from build123d import *

# Parameters (mm, degrees)
F1_DEPTH = 25.4
F2_R     = 3.175
F3_DEPTH = 25.4
F4_T     = -2.54


with BuildPart() as f1:
    # F0 (on Front) → F1 (new body)
    with BuildSketch(Plane.XZ):
        with BuildLine():
            Line((-63.5, -38.1), (63.5, -38.1))
            Line((63.5, -38.1), (63.5, 3.0236337334))
            Line((63.5, 3.0236337334), (6.35, 38.1))
            Line((6.35, 38.1), (-50.8, 38.1))
            ThreePointArc((-50.8, 38.1), (-59.7802561211, 34.3802561211), (-63.5, 25.4))
            Line((-63.5, 25.4), (-63.5, -38.1))
        make_face()
    extrude(amount=F1_DEPTH)

    # F2 (on face) → F3 (cut)
    with BuildSketch(Plane.XZ.offset(25.4)):
        with Locations((-50.8, 25.4)):
            Circle(F2_R)
        with Locations((-50.8, 0)):
            Circle(F2_R)
        with Locations((-50.8, -25.4)):
            Circle(F2_R)
        with Locations((-38.1, 25.4)):
            Circle(F2_R)
        with Locations((-38.1, 0)):
            Circle(F2_R)
        with Locations((-38.1, -25.4)):
            Circle(F2_R)
        with Locations((-25.4, 25.4)):
            Circle(F2_R)
        with Locations((-25.4, 0)):
            Circle(F2_R)
        with Locations((-25.4, -25.4)):
            Circle(F2_R)
        with Locations((-12.7, 25.4)):
            Circle(F2_R)
        with Locations((-12.7, 0)):
            Circle(F2_R)
        with Locations((-12.7, -25.4)):
            Circle(F2_R)
        with Locations((25.4, 0)):
            Circle(F2_R)
        with Locations((50.8, -25.4)):
            Circle(F2_R)
        with Locations((38.1, -25.4)):
            Circle(F2_R)
        with Locations((12.7, 0)):
            Circle(F2_R)
        with Locations((50.8, 25.4)):
            Circle(F2_R)
        with Locations((38.1, 25.4)):
            Circle(F2_R)
        with Locations((25.4, 25.4)):
            Circle(F2_R)
        with Locations((12.7, 25.4)):
            Circle(F2_R)
        with Locations((38.1, 0)):
            Circle(F2_R)
        with Locations((50.8, 0)):
            Circle(F2_R)
        with Locations((25.4, -25.4)):
            Circle(F2_R)
        with Locations((12.7, -25.4)):
            Circle(F2_R)
    extrude(amount=-F3_DEPTH, mode=Mode.SUBTRACT)

    # F4
    f4_openings = [f1.faces().sort_by_distance(p)[0] for p in [
        (-4.94859, 0, -3.243441),
    ]]
    offset(amount=F4_T, openings=f4_openings, kind=Kind.INTERSECTION)


solid = f1.part
CAD build for the part. Positions are in the model's coordinates, mm. A direction names the side the tool comes from. Coordinates: 2 decimals unless noted, no trailing zeros. Write each loop counter-clockwise with the first axis right and the second up, starting at its lowest first coordinate (ties: lowest second). Pieces come first, ordered by that corner, then holes. Notation, with made-up numbers: M 74,-35 L 101,-35 A31 cw 101,-7 Z; hole C 89.25,43 d6. An arc over 180 degrees is marked long. Return JSON: item names as keys, results as strings.
Item 1: Drop flat-ended pins along their axis: pin 1 Ø5.5 at (x, z) = (-38.1, 25.4) entering from -Y; pin 2 Ø1.5 at (x, z) = (10, -16) entering from +Y; pin 3 Ø2 at (x, y) = (28.5, -17.5) entering from +Z. Give the stop position or say it passes through.
Findings below:
{"pin 1": "passes through", "pin 2": "stops at y = -22.86", "pin 3": "stops at z = 24.53"}
Item 2: Which spindle directions (+Z, -Z, +X, -X, +Y, -Y) get a long thin tool onto all of the face, cutting with end or side? Do faces 1 (the flat face through (-60.96, -11, -5)), 2 (the flat face through (63.5, -13, -18)). Say none if no direction does.
Findings below:
{"face 1": "+Y", "face 2": "+Z, -Z, +X, +Y, -Y"}
Item 3: Slice it at C-C, the plane x = 38.1. Write the cut outline in (y, z) (3 decimals), and give its area (3 significant figures).
Findings below:
{"outline": "M -25.4,-38.1 L 0,-38.1 L 0,-35.56 L -22.86,-35.56 L -22.86,-31.115 L 0,-31.115 L 0,-28.575 L -25.4,-28.575 Z; M -25.4,-22.225 L 0,-22.225 L 0,-19.685 L -22.86,-19.685 L -22.86,-5.715 L 0,-5.715 L 0,-3.175 L -25.4,-3.175 Z; M -25.4,3.175 L 0,3.175 L 0,5.715 L -22.86,5.715 L -22.86,15.633 L 0,15.633 L 0,18.613 L -25.4,18.613 Z", "area": "470 mm2"}
Item 4: Two-plate mould, pull along Z, no slides. Class faces 3 (the flat face through (45.29, -11.27, 11.22)), 4 (the flat face through (15.2, 0, -2.5)): +Z half, -Z half, draft (parallel to the pull), parting line (faces both ways), or undercut.
Findings below:
{"face 3": "undercut", "face 4": "draft"}
Item 5: Probe line 1 (Z direction, x = -4, y = -10.5); line 2 (X direction, y = -5, z = -13.5); line 3 (Z direction, x = -16, y = -15.5). List the from-to ranges inside material, lowest first. Write a range as from..to.
Findings below:
{"line 1": "z = -38.1..-35.56, 35.56..38.1", "line 2": "x = -63.5..-60.96, 60.96..63.5", "line 3": "z = -38.1..-35.56, -30.07..-20.73, -4.67..4.67, 20.73..30.07, 35.56..38.1"}
Item 6: Slice it at A-A, the plane x = -38.1. State how many separate pieces and enclosed holes the cut face has, and give its area (3 significant figures).
Findings below:
{"separate pieces": "4", "enclosed holes": "0", "area": "610 mm2"}
